Verification items for this drawing (mm, ordinates from the low corner). A direction names the side the tool comes from. Coordinates: 2 decimals unless noted, no trailing zeros. Order: outer loops, then holes, each group sorted by start corner. A loop starts at its lowest first (then second) coordinate and runs counter-clockwise, first axis right, second up. Notation, with made-up numbers: (83, -38.5) -> (118, -38.5) arc R25 cw to (118, -4.5) -> close; hole circle Ø3 at (12, -2). An arc over 180 degrees is marked (long way). Write each question's results on one line, items separated by ' | '. Start each with the question number.
(1) Cross-section at C-C on z = 5.5. Enter the section's corners in (x, y), and give its area (3 significant figures).
(2) Set-up check for the marked faces 1, 2 and 3: record each of +Z, -Z, +X, -X, +Y, -Y from which the full face is reachable in a straight line by a thin tool's end or side.
(3) Thickness scan on probe 1 along X at (y, z) = (29.5, 13); probe 2 along X at (y, z) = (30, 23.25); probe 3 along Y at (x, z) = (131, 4). Record the ranges inside material, lowest first. Write a range as [from, to].
(4) Go/stop test with flat-tipped pins: pin 1 (9.5 mm diameter, centred on x = 146, z = 19, fed in from +Y); pin 2 (7.5 mm diameter, centred on y = 15.5, z = 12.5, fed in from +X); pin 3 (11.5 mm diameter, centred on x = 104.5, y = 37, fed in from +Z). Record where each tip stops, or that it passes through.
(5) Cross-section at B-B on z = 11.25. Enter the section's corners in (x, y).
(6) Cross-section at A-A on y = 38. Enter the section's corners in (x, z).
(7) Cross-section at D-D on y = 24.5. Enter the section's corners in (x, z), and give its area (3 significant figures).
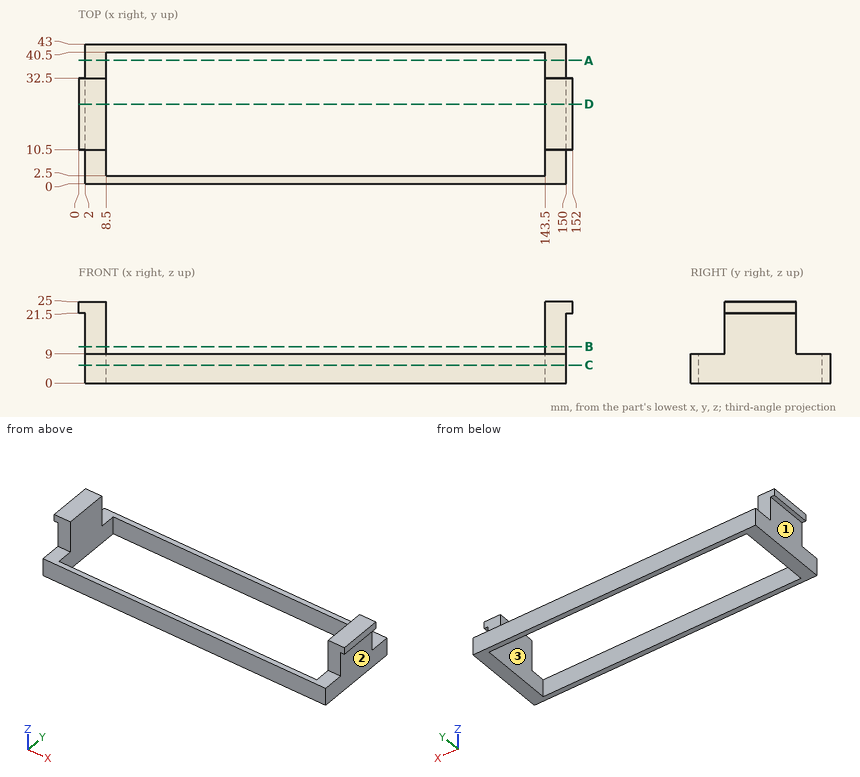
Results are:
1) outline: (2, 0) -> (150, 0) -> (150, 43) -> (2, 43) -> close; hole (8.5, 2.5) -> (143.5, 2.5) -> (143.5, 40.5) -> (8.5, 40.5) -> close | area: 1,230 mm2
2) face 1: -Z, -X, +Y, -Y | face 2: -Z, +X, +Y, -Y | face 3: +Z, -Z
3) probe 1: x = [2, 8.5], [143.5, 150] | probe 2: x = [0, 8.5], [143.5, 152] | probe 3: y = [0, 2.5], [40.5, 43]
4) pin 1: stops at y = 32.5 | pin 2: stops at x = 150 | pin 3: stops at z = 9
5) outline: (2, 10.5) -> (8.5, 10.5) -> (8.5, 32.5) -> (2, 32.5) -> close; (143.5, 10.5) -> (150, 10.5) -> (150, 32.5) -> (143.5, 32.5) -> close
6) outline: (2, 0) -> (8.5, 0) -> (8.5, 9) -> (2, 9) -> close; (143.5, 0) -> (150, 0) -> (150, 9) -> (143.5, 9) -> close
7) outline: (0, 21.5) -> (2, 21.5) -> (2, 0) -> (8.5, 0) -> (8.5, 25) -> (0, 25) -> close; (143.5, 0) -> (150, 0) -> (150, 21.5) -> (152, 21.5) -> (152, 25) -> (143.5, 25) -> close | area: 339 mm2
